The listing builds one solid part. Answer for the finished solid, in the listing's coordinates (mm). Give positions to 0.01 mm unless a question says otherwise; leave off trailing zeros. Order: outer loops, then holes, each group sorted by start corner. A loop starts at its lowest first (then second) coordinate and runs counter-clockwise, first axis right, second up. Notation, with made-up numbers: (-30.5, -13) - (28.5, -13) arc R18 cw to (28.5, 12) - close; hole circle Ø3 at (-7.5, 70.25). An arc over 180 degrees is marked (long way). Answer as CSV lines item,"result". Start each with the question number.
1. Flat-ended cylindrical pins translate along their axes: pin 1 (5 mm diameter, centred on x = 8.5, y = 7, fed in from +Z); pin 2 (2 mm diameter, centred on x = 9, y = 10.5, fed in from +Z). Find the tip coordinate at first contact, or state that the pin passes through.
2. Section D-D on y = 14.75 is taken. Give the vertices of the cut face in (x, z), and give its area (3 significant figures).
3. Section A-A on z = -6.35 is taken. Count the separate pieces of the cut face and the enclosed holes in it, and give its area (3 significant figures).
4. Consider line 1 along X through (y, z) = (13.25, -66.04); line 2 along Z through (x, y) = (6.35, 5); line 3 along Z through (x, y) = (6.35, 4.5). Determine where each line is inside the solid, lowest interval first. Write a range as [from, to].
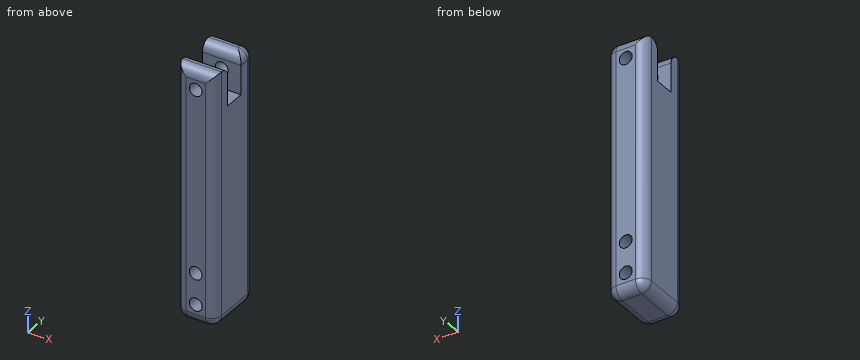
Autodesk Inventor part; units mm, degrees
ref_plane "YZ Plane" through (0, 0, 0) normal (1, 0, 0) x (0, 1, 0)
ref_plane "XZ Plane" through (0, 0, 0) normal (0, 1, 0) x (-1, 0, 0)
ref_plane "XY Plane" through (0, 0, 0) normal (0, 0, 1) x (1, 0, 0)
sketch "Sketch1" plane through (0, 0, 0) normal (1, 0, 0) x (0, 1, 0)
  line L0 (0, 0) -> (6.35, 0)
  line L1 (6.35, 0) -> (6.35, -12.7)
  line L2 (6.35, -12.7) -> (13.081, -12.7)
  line L3 (13.081, -12.7) -> (13.081, 0)
  line L4 (13.081, 0) -> (19.431, 0)
  line L5 (19.431, 0) -> (19.431, -82.55)
  line L6 (19.431, -82.55) -> (0, -82.55)
  line L7 (0, -82.55) -> (0, 0)
  dimension "d0" = 6.35
  dimension "d1" = 12.7
  dimension "d2" = 6.731
  dimension "d11" = 6.35
  dimension "d12" = 82.55
  dimension "d18" = 12.7
extrude "Extrusion1" add sketch "Sketch1" along normal blind 12.7
sketch "Sketch3" plane through (0, 19.431, 0) normal (0, 1, 0) x (1, 0, 0)
  line L0 (0, 12.7) -> (12.7, 12.7)
  line L1 (12.7, 12.7) -> (0, 12.7)
  line L2 (0, 12.7) -> (0, 0)
  line L3 (0, 0) -> (12.7, 0)
  line L4 (12.7, 0) -> (12.7, 12.7)
  line L5 (0, 0) -> (12.7, 12.7)
  circle A0 centre (6.35, 6.35) radius 2.1082
  line L6 (0, 82.55) -> (12.7, 82.55)
  line L7 (6.35, 82.55) -> (6.35, 76.2)
  circle A1 centre (6.35, 76.2) radius 2.1082
  dimension "d13" = 4.2164
  dimension "d16" = 6.35
  dimension "d17" = 4.2164
extrude "Extrusion3" cut sketch "Sketch3" against normal blind 28.575 contours A0 L5 | L5 A0 | A1
fillet "Fillet1" radius 3.175 1 edges at (12.7, 19.431, -41.275)
fillet "Fillet2" radius 3.175 14 edges at (11.7701, 18.5011, 0) (12.7, 14.6685, 0) (4.7625, 19.431, 0) (0, 19.431, -41.275) (11.7701, 18.5011, -82.55) (12.7, 8.128, -82.55) (4.7625, 19.431, -82.55) (0, 9.7155, -82.55) (12.7, 0, -41.275) (6.35, 0, -82.55) (0, 0, -41.275) (6.35, 0, 0) (6.35, 6.35, 0) (6.35, 13.081, 0)
sketch "Sketch5" plane through (3.175, 19.431, -3.175) normal (0, 1, 0) x (1, 0, 0)
  circle A0 centre (3.175, 73.025) radius 2.1082
  line L0 (3.175, 73.025) -> (3.175, 62.865)
  circle A1 centre (3.175, 62.865) radius 2.1082
  point P0 (-3.175, -3.175)
  dimension "d26" = 10.16
extrude "Extrusion5" cut sketch "Sketch5" against normal blind 25.4 contours A1
properties part number "wing bar"
Checks:
1,pin 1,"stops at z = -0.29"
1,pin 2,"stops at z = -12.7"
2,outline,"(0, -79.38) arc R3.17 ccw to (3.17, -82.55) - (9.53, -82.55) arc R3.17 ccw to (12.7, -79.38) - (12.7, -3.17) arc R3.17 ccw to (11.03, -0.38) - (0, -0.38) - close; hole circle Ø4.22 at (6.35, -76.2); hole circle Ø4.22 at (6.35, -66.04); hole circle Ø4.22 at (6.35, -6.35)"
2,area,"996 mm²"
3,separate pieces,"4"
3,enclosed holes,"0"
3,area,"99.1 mm²"
4,line 1,"x = [0, 4.24], [8.46, 12.7]"
4,line 2,"z = [-82.55, -78.31], [-74.09, -68.15], [-63.93, -8.46], [-4.24, -0.58]"
4,line 3,"z = [-82.55, -78.31], [-74.09, -68.15], [-63.93, -8.46], [-4.24, -0.29]"
